Could you check a few things on this model? Use its own coordinates, in mm. Coordinates: 2 decimals unless noted, no trailing zeros. Loops run counter-clockwise (first coordinate to the right, second up) from the corner with the lowest first, then second, coordinate; pieces in that order, holes last. Notation, with made-up numbers: M 70.25,26 L 75.25,26 A16 cw 75.25,46 Z; hole C 51,53.5 d11. An arc over 180 degrees is marked long. Write each question's results on one line, items separated by ' | '.
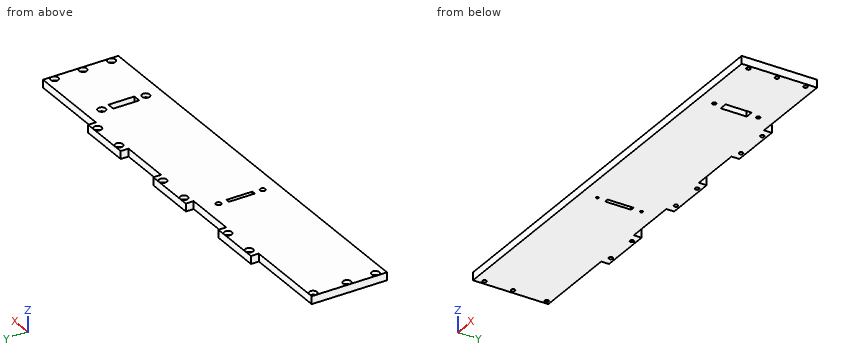
```python
from build123d import *

# Parameters (mm, degrees)
ESQUISSE1_W             = 330
ESQUISSE1_H             = 64
BOSS_EXTRU_1_DEPTH      = 6
ESQUISSE2_W             = 65
ESQUISSE2_H             = 6
ESQUISSE2_W_2           = 40
ENL_V_MAT_EXTRU_1_DEPTH = 337.20232004
ESQUISSE3_W             = 3
ESQUISSE3_H             = 20
ESQUISSE3_W_2           = 6
ENL_V_MAT_EXTRU_2_DEPTH = 337.20232004
ESQUISSE4_R             = 1.5
ESQUISSE4_R_2           = 1.005
ENL_V_MAT_EXTRU_3_DEPTH = 337.20232004
ESQUISSE5_R             = 2.995
ESQUISSE5_R_2           = 2
ENL_V_MAT_EXTRU_4_DEPTH = 3


with BuildPart() as part:
    # Esquisse1 → Boss.-Extru.1 (new body)
    with BuildSketch(Plane.XY):
        with Locations((-165, 32)):
            Rectangle(ESQUISSE1_W, ESQUISSE1_H)
    extrude(amount=BOSS_EXTRU_1_DEPTH)

    # Esquisse2 → Enlèv. mat.-Extru.1 (cut, through all)
    with BuildSketch(Plane.XY.offset(6)):
        with Locations((-297.5, 61)):
            Rectangle(ESQUISSE2_W, ESQUISSE2_H)
        with Locations((-205, 61)):
            Rectangle(ESQUISSE2_W_2, ESQUISSE2_H)
        with Locations((-125, 61)):
            Rectangle(ESQUISSE2_W_2, ESQUISSE2_H)
        with Locations((-32.5, 61)):
            Rectangle(ESQUISSE2_W, ESQUISSE2_H)
    extrude(amount=-ENL_V_MAT_EXTRU_1_DEPTH, mode=Mode.SUBTRACT)

    # Esquisse3 → Enlèv. mat.-Extru.2 (cut, through all)
    with BuildSketch(Plane.XY.offset(6)):
        with Locations((-196.5, 29)):
            Rectangle(ESQUISSE3_W, ESQUISSE3_H)
        with Locations((-53, 29)):
            Rectangle(ESQUISSE3_W_2, ESQUISSE3_H)
    extrude(amount=-ENL_V_MAT_EXTRU_2_DEPTH, mode=Mode.SUBTRACT)

    # Esquisse4 → Enlèv. mat.-Extru.3 (cut, through all)
    with BuildSketch(Plane.XY.offset(6)):
        with Locations((-327, 55)):
            Circle(ESQUISSE4_R)
        with Locations((-327, 29)):
            Circle(ESQUISSE4_R)
        with Locations((-327, 7)):
            Circle(ESQUISSE4_R)
        with Locations((-258, 61)):
            Circle(ESQUISSE4_R)
        with Locations((-232, 61)):
            Circle(ESQUISSE4_R)
        with Locations((-178, 61)):
            Circle(ESQUISSE4_R)
        with Locations((-152, 61)):
            Circle(ESQUISSE4_R)
        with Locations((-98, 61)):
            Circle(ESQUISSE4_R)
        with Locations((-72, 61)):
            Circle(ESQUISSE4_R)
        with Locations((-53, 46)):
            Circle(ESQUISSE4_R)
        with Locations((-53, 12)):
            Circle(ESQUISSE4_R)
        with Locations((-196.5, 46)):
            Circle(ESQUISSE4_R_2)
        with Locations((-196.5, 12)):
            Circle(ESQUISSE4_R_2)
        with Locations((-3, 51)):
            Circle(ESQUISSE4_R)
        with Locations((-3, 29)):
            Circle(ESQUISSE4_R)
        with Locations((-3, 7)):
            Circle(ESQUISSE4_R)
    extrude(amount=-ENL_V_MAT_EXTRU_3_DEPTH, mode=Mode.SUBTRACT)

    # Esquisse5 → Enlèv. mat.-Extru.4 (cut)
    with BuildSketch(Plane.XY.offset(6)):
        with Locations((-327, 7)):
            Circle(ESQUISSE5_R)
        with Locations((-327, 29)):
            Circle(ESQUISSE5_R)
        with Locations((-327, 55)):
            Circle(ESQUISSE5_R)
        with Locations((-258, 61)):
            Circle(ESQUISSE5_R)
        with Locations((-232, 61)):
            Circle(ESQUISSE5_R)
        with Locations((-196.5, 46)):
            Circle(ESQUISSE5_R_2)
        with Locations((-178, 61)):
            Circle(ESQUISSE5_R)
        with Locations((-152, 61)):
            Circle(ESQUISSE5_R)
        with Locations((-98, 61)):
            Circle(ESQUISSE5_R)
        with Locations((-72, 61)):
            Circle(ESQUISSE5_R)
        with Locations((-53, 46)):
            Circle(ESQUISSE5_R)
        with Locations((-53, 12)):
            Circle(ESQUISSE5_R)
        with Locations((-3, 7)):
            Circle(ESQUISSE5_R)
        with Locations((-3, 29)):
            Circle(ESQUISSE5_R)
        with Locations((-3, 51)):
            Circle(ESQUISSE5_R)
        with Locations((-196.5, 12)):
            Circle(ESQUISSE5_R_2)
    extrude(amount=-ENL_V_MAT_EXTRU_4_DEPTH, mode=Mode.SUBTRACT)


solid = part.part
```
(1) Imagine slicing it at C-C, the plane x = -202.5. List the corners of the cut face in (y, z) for me.
Reported:
outline: M 0,0 L 58,0 L 58,6 L 0,6 Z
(2) Imagine slicing it at A-A, the plane y = 22.5. List the corners of the cut face in (x, z) for me, and give its area (3 significant figures).
Reported:
outline: M -330,0 L -198,0 L -198,6 L -330,6 Z; M -195,0 L -56,0 L -56,6 L -195,6 Z; M -50,0 L 0,0 L 0,6 L -50,6 Z | area: 1,930 mm2
(3) Imagine slicing it at B-B, the plane z = 1.6. State how many separate pieces and enclosed holes the cut face has, and give its area (3 significant figures).
Reported:
separate pieces: 1 | enclosed holes: 18 | area: 19,600 mm2
(4) Please list where these lines run through material, in increasing order: probe 1 along Y at (x, z) = (-3, 5) (3 decimals); probe 2 along Y at (x, z) = (-3, 1.5); probe 3 along Y at (x, z) = (-72, 0.7). Write a range as from..to.
Reported:
probe 1: y = 0..4.005, 9.995..26.005, 31.995..48.005, 53.995..58 | probe 2: y = 0..5.5, 8.5..27.5, 30.5..49.5, 52.5..58 | probe 3: y = 0..59.5, 62.5..64
(5) Will these pins go through, and if not, where does the flat tip stop? P1, Ø3, axis at y = 60, z = 3, coming from the -X side; P2, Ø3, axis at x = -53.5, y = 13, coming from the +Z side; P3, Ø2.5, axis at x = -3, y = 7, coming from the -Z side; P4, Ø3, axis at x = -290, z = 4, coming from the +Y side.
Reported:
P1: stops at x = -265 | P2: stops at z = 3 | P3: passes through | P4: stops at y = 58
